```python
from build123d import *

# Parameters (mm, degrees)
F0_R     = 1.75
F1_DEPTH = 25
F2_DEPTH = 24


with BuildPart() as f1:
    # F0 (on Top) → F1 (new body)
    with BuildSketch(Plane.XY):
        with BuildLine():
            Line((6.5, -12.5), (12.5, -12.5))
            Line((12.5, -12.5), (12.5, 12.5))
            Line((12.5, 12.5), (-12.5, 12.5))
            Line((-12.5, 12.5), (-12.5, -12.5))
            Line((-12.5, -12.5), (-6.5, -12.5))
            Line((-6.5, -12.5), (-6.5, -7.5993420768))
            ThreePointArc((-6.5, -7.5993420768), (-4.1833001327, 9.0829510623), (10, 0))
            ThreePointArc((10, 0), (9.0829510623, -4.1833001327), (6.5, -7.5993420768))
            Line((6.5, -7.5993420768), (6.5, -12.5))
        make_face()
        with Locations((-9, -9)):
            Circle(F0_R, mode=Mode.SUBTRACT)
        with Locations((9, -9)):
            Circle(F0_R, mode=Mode.SUBTRACT)
        with BuildLine():
            ThreePointArc((-6.5, -7.5993420768), (0, -10), (6.5, -7.5993420768))
            ThreePointArc((6.5, -7.5993420768), (9.0829510623, -4.1833001327), (10, 0))
            ThreePointArc((10, 0), (-4.1833001327, 9.0829510623), (-6.5, -7.5993420768))
        make_face()
        Circle(F0_R, mode=Mode.SUBTRACT)
    extrude(amount=F1_DEPTH)

    # F0 (on Top) → F2 (cut)
    with BuildSketch(Plane.XY):
        with BuildLine():
            ThreePointArc((-6.5, -7.5993420768), (0, -10), (6.5, -7.5993420768))
            ThreePointArc((6.5, -7.5993420768), (9.0829510623, -4.1833001327), (10, 0))
            ThreePointArc((10, 0), (-4.1833001327, 9.0829510623), (-6.5, -7.5993420768))
        make_face()
        Circle(F0_R, mode=Mode.SUBTRACT)
    extrude(amount=F2_DEPTH, mode=Mode.SUBTRACT)


solid = f1.part
```
For this review, take the finished solid that the model builds, in its own axes (mm). A direction names the side the tool comes from. Round coordinates to 2 decimals unless told otherwise and drop trailing zeros. Write each loop counter-clockwise with the first axis right and the second up, starting at its lowest first coordinate (ties: lowest second). Pieces come first, ordered by that corner, then holes. Notation, with made-up numbers: (-35.5, -3.5) - (23.5, -3.5) arc R30 cw to (23.5, 25.5) - close; hole circle Ø2 at (36.25, 14). An arc over 180 degrees is marked (long way). Use CSV: the item, a comma, the result in double quotes.
1) The part is to be moulded in two halves that separate along X. For faces 1 (the flat face through (12.5, 0, 12)), 2 (the cylindrical face through (1.617, -0.67, 24.493)), 3 (the flat face through (9, -12.5, 12)), say which applies: pulls with the +X half, pulls with the -X half, needs draft (parallel to the pull), parting line crosses it, or undercut.
Conclusion:
face 1,"pulls with the +X half"
face 2,"undercut"
face 3,"needs draft"
2) Add section D-D on x = -8.75. Write out the cut boundary in (y, z).
Conclusion:
outline,"(-12.5, 0) - (-10.73, 0) - (-10.73, 25) - (-12.5, 25) - close; (-7.27, 0) - (-4.84, 0) - (-4.84, 24) - (4.84, 24) - (4.84, 0) - (12.5, 0) - (12.5, 25) - (-7.27, 25) - close"
3) Wall thickness on line 1 along X through (y, z) = (0, 19); line 2 along Y through (x, z) = (-9, 12.25); line 3 along Z through (x, y) = (-6, -1.75): over which ranges is each line inside the solid? List them lowest first. Write a range as from..to.
Conclusion:
line 1,"x = -12.5..-10, 10..12.5"
line 2,"y = -12.5..-10.75, -7.25..-4.36, 4.36..12.5"
line 3,"z = 24..25"
4) Clearance check with a flat-ended pin moving along its axis: pin 1 Ø1.5 at (x, y) = (6.5, -1) entering from -Z. State where the tip first meets the part, or that it passes through.
Conclusion:
pin 1,"stops at z = 24"
5) For faces 4 (the flat face through (6.5, -10, 12)), 5 (the flat face through (0, -2, 24)), 6 (the flat face through (-10, -12.5, 12)), list the 3-axis set-ups (+Z, -Z, +X, -X, +Y, -Y) from which the entire face can be reached by the end or side of a thin tool; tool diameter is ignored.
Conclusion:
face 4,"+Z, -Z, -Y"
face 5,"-Z"
face 6,"+Z, -Z, +X, -X, -Y"
6) Add section C-C on y = -9. Write out the cut boundary in (x, z), and give its area (3 significant figures).
Conclusion:
outline,"(-12.5, 0) - (-10.75, 0) - (-10.75, 25) - (-12.5, 25) - close; (-7.25, 0) - (-6.5, 0) - (-6.5, 25) - (-7.25, 25) - close; (-4.36, 24) - (4.36, 24) - (4.36, 25) - (-4.36, 25) - close; (6.5, 0) - (7.25, 0) - (7.25, 25) - (6.5, 25) - close; (10.75, 0) - (12.5, 0) - (12.5, 25) - (10.75, 25) - close"
area,"134 mm^2"
7) Add section A-A on z = 10.75. Write out the cut boundary in (x, y), and give its area (3 significant figures).
Conclusion:
outline,"(-12.5, -12.5) - (-6.5, -12.5) - (-6.5, -7.6) arc R10 cw (long way) to (6.5, -7.6) - (6.5, -12.5) - (12.5, -12.5) - (12.5, 12.5) - (-12.5, 12.5) - close; hole circle Ø3.5 at (-9, -9); hole circle Ø3.5 at (9, -9)"
area,"249 mm^2"
8) Add section B-B on x = 0. Write out the cut boundary in (y, z).
Conclusion:
outline,"(-10, 24) - (-1.75, 24) - (-1.75, 25) - (-10, 25) - close; (1.75, 24) - (10, 24) - (10, 0) - (12.5, 0) - (12.5, 25) - (1.75, 25) - close"
